```python
from build123d import *

# Parameters (mm, degrees)
ESBO_O1_R                = 28.7
RESSALTO_EXTRUS_O1_DEPTH = 5
ESBO_O2_R                = 11
CORTE_EXTRUS_O1_DEPTH    = 8
ESBO_O3_R                = 7.5
CORTE_EXTRUS_O2_DEPTH    = 42.801674608
RESSALTO_EXTRUS_O4_START = 10
RESSALTO_EXTRUS_O4_DEPTH = 10
ESBO_O9_W                = 10
ESBO_O9_H                = 2
CORTE_EXTRUS_O5_DEPTH    = 10
CHANFRO1_SIZE            = 2
ESBO_O10_R               = 1.8
CORTE_EXTRUS_O6_DEPTH    = 10
CORTE_EXTRUS_O7_START    = -3
CORTE_EXTRUS_O7_DEPTH    = 2.9


with BuildPart() as part:
    # Esboço1 → Ressalto-extrusão1 (new, symmetric)
    with BuildSketch(Plane.XY):
        Circle(ESBO_O1_R)
    extrude(amount=RESSALTO_EXTRUS_O1_DEPTH, both=True)

    # Esboço2 → Corte-extrusão1 (cut)
    with BuildSketch(Plane.XY.offset(5)):
        Circle(ESBO_O2_R)
    extrude(amount=-CORTE_EXTRUS_O1_DEPTH, mode=Mode.SUBTRACT)

    # Esboço3 → Corte-extrusão2 (cut, through all)
    with BuildSketch(Plane(origin=(0, 0, -5), x_dir=(-1, 0, 0), z_dir=(0, 0, -1))):
        Circle(ESBO_O3_R)
    extrude(amount=-CORTE_EXTRUS_O2_DEPTH, mode=Mode.SUBTRACT)

    # Esboço8 → Ressalto-extrusão4 (add)
    with BuildSketch(Plane.XY.offset(5).offset(RESSALTO_EXTRUS_O4_START)):
        with BuildLine():
            Line((-11, 0), (-28.7, 0))
            ThreePointArc((-28.7, 0), (0, -28.7), (28.7, 0))
            Line((28.7, 0), (11, 0))
            ThreePointArc((11, 0), (0, -11), (-11, 0))
        make_face()
    extrude(amount=-RESSALTO_EXTRUS_O4_DEPTH)

    # Esboço9 → Corte-extrusão5 (cut)
    with BuildSketch(Plane.XY.offset(15)):
        with Locations((-19.85, -1)):
            Rectangle(ESBO_O9_W, ESBO_O9_H)
        with Locations((19.85, -1)):
            Rectangle(ESBO_O9_W, ESBO_O9_H)
    extrude(amount=-CORTE_EXTRUS_O5_DEPTH, mode=Mode.SUBTRACT)

    # Chanfro1
    chanfro1_edges = [part.edges().sort_by_distance(p)[0] for p in [
        (24.85, 0, 10),
        (14.85, 0, 10),
        (-14.85, 0, 10),
        (-24.85, 0, 10),
    ]]
    chamfer(chanfro1_edges, length=CHANFRO1_SIZE - 0.0001)  # a hair under: the kernel refuses the full size

    # Esboço10 → Corte-extrusão6 (cut)
    with BuildSketch(Plane(origin=(0, -2, 0), x_dir=(1, 0, 0), z_dir=(0, 1, 0))):
        with Locations(Location((-19.85, -10, 0), (0, 0, 180))):
            Circle(ESBO_O10_R)
        with Locations((19.85, -10)):
            Circle(ESBO_O10_R)
    extrude(amount=-CORTE_EXTRUS_O6_DEPTH, mode=Mode.SUBTRACT)

    # Esboço11 → Corte-extrusão7 (cut)
    with BuildSketch(Plane(origin=(0, -2, 0), x_dir=(1, 0, 0), z_dir=(0, 1, 0)).offset(CORTE_EXTRUS_O7_START)):
        Polygon((-23, -8.181346652), (-23, -11.818653348), (-23, -15), (-16.7, -15), (-16.7, -11.818653348), (-16.7, -8.181346652), (-19.85, -6.362693304), align=None)
        Polygon((23, -15), (23, -11.818653348), (23, -8.181346652), (19.85, -6.362693304), (16.7, -8.181346652), (16.7, -11.818653348), (16.7, -15), align=None)
    extrude(amount=-CORTE_EXTRUS_O7_DEPTH, mode=Mode.SUBTRACT)


solid = part.part
```
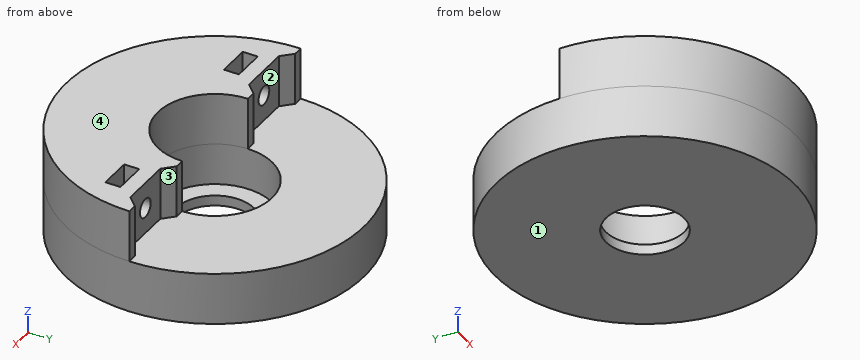
Verification items for the finished model (mm, model axes). Face numbers are marked on the shaded views. A direction names the side the tool comes from. Coordinates: 2 decimals unless noted, no trailing zeros. Order: outer loops, then holes, each group sorted by start corner. A loop starts at its lowest first (then second) coordinate and runs counter-clockwise, first axis right, second up. Notation, with made-up numbers: (9.5, 62.25) -> (66.5, 62.25) arc R26 cw to (66.5, 83.25) -> close; hole circle Ø6 at (-25, -18). An arc over 180 degrees is marked (long way). Answer as CSV lines item,"result". Start each with the question number.
1) Material ranges on L1, parallel to Z at x = -19.85, y = -3.1; L2, parallel to Z at x = -15, y = 24; L3, parallel to Z at x = 9, y = 0.5, recorded low to high. Write a range as [from, to].
2) Release check for a two-part mould opening along X. For the marked faces 3 and 4 record: released by +X, released by -X, zero draft, split by the parting line, or undercut.
3) Gauge pin test, flat ends, axial feed: pin 1 Ø1 at (y, z) = (19.5, 4.5) entering from -X; pin 2 Ø3 at (x, z) = (-19, 9.5) entering from +Y; pin 3 Ø8 at (y, z) = (-18.5, 8.5) entering from -X. Record the tip position at first contact, or that the pin passes through.
4) Cross-section at D-D, the plane y = 15. Record the boundary of the cut face in (x, z).
5) Cross-section at A-A, the plane x = 0. Record the boundary of the cut face in (y, z), then the cut area to 3 significant figures.
6) Cross-section at B-B, the plane z = -1.75. Record the boundary of the cut face in (x, y), then the cut area to 3 significant figures.
7) Cross-section at C-C, the plane x = 10. Record the boundary of the cut face in (y, z), then the cut area to 3 significant figures.
8) Set-up check for the marked faces 1 and 2: record each of +Z, -Z, +X, -X, +Y, -Y from which the full face is reachable in a straight line by a thin tool's end or side.
Conclusion:
1,L1,"z = [-5, 8.2], [11.8, 15]"
1,L2,"z = [-5, 5]"
1,L3,"z = [-5, -3]"
2,face 3,"undercut"
2,face 4,"zero draft"
3,pin 1,"stops at x = -21.51"
3,pin 2,"stops at y = -2"
3,pin 3,"stops at x = -24.77"
4,outline,"(-24.47, -5) -> (24.47, -5) -> (24.47, 5) -> (-24.47, 5) -> close"
5,outline,"(-28.7, -5) -> (-7.5, -5) -> (-7.5, -3) -> (-11, -3) -> (-11, 15) -> (-28.7, 15) -> close; (7.5, -5) -> (28.7, -5) -> (28.7, 5) -> (11, 5) -> (11, -3) -> (7.5, -3) -> close"
5,area,"545 mm²"
6,outline,"circle Ø57.4 at (0, 0); hole circle Ø22 at (0, 0)"
6,area,"2,210 mm²"
7,outline,"(-26.9, -5) -> (26.9, -5) -> (26.9, 5) -> (4.58, 5) -> (4.58, -3) -> (-4.58, -3) -> (-4.58, 15) -> (-26.9, 15) -> close"
7,area,"688 mm²"
8,face 1,"-Z, +X, -X, +Y, -Y"
8,face 2,"+Z, +Y"
